Autodesk Inventor part; units mm, degrees
ref_plane "YZ Plane" through (0, 0, 0) normal (1, 0, 0) x (0, 1, 0)
ref_plane "XZ Plane" through (0, 0, 0) normal (0, 1, 0) x (-1, 0, 0)
ref_plane "XY Plane" through (0, 0, 0) normal (0, 0, 1) x (1, 0, 0)
sketch "Boceto1" plane through (0, 0, 0) normal (0, 0, 1) x (1, 0, 0)
  line L0 (0, 50.8) -> (-20.2, 50.8)
  line L1 (-20.2, 50.8) -> (-20.2, 0)
  line L2 (-20.2, 0) -> (0, 0)
  line L3 (0, 0) -> (0, 50.8)
  dimension "d0" = 50.8
  dimension "d1" = 20.2
extrude "Extrusión1" add sketch "Boceto1" against normal blind 3.4
sketch "Boceto3" plane through (0, 0, 0) normal (0, 0, -1) x (-1, 0, 0)
  line L0 (20.2, 50.8) -> (0, 50.8) construction
  line L1 (0, 50.8) -> (0, 0) construction
  circle A0 centre (10.1, 42.1) radius 2
  line L2 (20.2, 0) -> (20.2, 50.8)
  dimension "d20" = 4
  dimension "d21" = 10.1
  dimension "d23" = 8.7
hole "Agujero3" at (-10.1, 42.1, 0) direction (0, 0, -1) diameter 4 end through all countersink diameter 6 countersink angle 90
sketch "Boceto5" plane through (0, 0, 0) normal (0, 0, -1) x (-1, 0, 0)
  line L0 (10.1, 29.1) -> (10.1, 22.1) construction
  line L1 (15.1, 29.1) -> (15.1, 22.1)
  line L2 (5.1, 22.1) -> (5.1, 29.1)
  arc A0 (15.1, 29.1) -> (5.1, 29.1) centre (10.1, 29.1) ccw
  arc A1 (5.1, 22.1) -> (15.1, 22.1) centre (10.1, 22.1) ccw
  circle A2 centre (10.1, 42.1) radius 3
  line L3 (0, 50.8) -> (0, 0)
  point P0 (10.1, 25.6)
  point P1 (10.1, 17.1)
  point P2 (10.1, 34.1)
  dimension "d31" = 10
  dimension "d32" = 17
  dimension "d34" = 5.1
extrude "Extrusión2" cut sketch "Boceto5" along normal through all contours L1 A1 L2 A0
sketch "Boceto6" plane through (0, 0, -3.4) normal (0, 0, -1) x (-1, 0, 0)
  line L0 (0, 0) -> (20.2, 0)
  line L1 (2.9, 0) -> (2.9, 12.8)
  line L2 (2.9, 12.8) -> (17.3, 12.8)
  line L3 (17.3, 12.8) -> (17.3, 0)
  line L4 (16, 0) -> (16, 11.5)
  line L5 (16, 11.5) -> (4.2, 11.5)
  line L6 (4.2, 11.5) -> (4.2, 0)
  line L7 (0, 50.8) -> (0, 0)
  line L8 (20.2, 0) -> (20.2, 50.8)
  point P0 (4.2, 0)
  point P1 (16, 0)
  dimension "d37" = 12.8
  dimension "d40" = 1.3
  dimension "d50" = 14.4
  dimension "d51" = 2.9
  dimension "d52" = 2.9
extrude "Extrusión3" add sketch "Boceto6" along normal blind 12.7 contours L1 L2 L3 L0 L4 L5 L6
sketch "Boceto7" plane through (0, 0, -3.4) normal (0, 0, -1) x (-1, 0, 0)
  line L0 (16, 11.5) -> (16, 0)
  line L1 (4.2, 11.5) -> (16, 11.5)
  line L2 (16, 11.5) -> (16, 0)
  line L3 (16, 0) -> (4.2, 0)
  line L4 (4.2, 0) -> (4.2, 11.5)
  point P0 (0, 0)
  point P1 (16, 11.5)
extrude "Extrusión4" cut sketch "Boceto7" against normal blind 10
properties part number "PLASTICO" material "Plástico ABS"
Input: part model. Units: mm. Frame: model coordinates. A direction names the side the tool comes from. Coordinates: 2 decimals unless noted, no trailing zeros. Order: outer loops, then holes, each group sorted by start corner. A loop starts at its lowest first (then second) coordinate and runs counter-clockwise, first axis right, second up. Notation, with made-up numbers: (44, 24.25) - (96, 24.25) arc R17 cw to (96, 32.25) - close; hole circle Ø2 at (13.5, 36). An arc over 180 degrees is marked (long way). Put each result on its own line as item: value.
1. Cut plane B-B on x = -10.1. Return the cut outline in (y, z).
Report:
outline: (11.5, -16.1) - (12.8, -16.1) - (12.8, -3.4) - (17.1, -3.4) - (17.1, 0) - (11.5, 0) - close; (34.1, -3.4) - (40.1, -3.4) - (40.1, -1) - (39.1, 0) - (34.1, 0) - close; (44.1, -3.4) - (50.8, -3.4) - (50.8, 0) - (45.1, 0) - (44.1, -1) - close
2. Draft query along Y for faces 5 (the face through (-10, 34.1, -1.7)), 6 (the face through (-17, 0, -6)), 7 (the face through (-4.2, 6, -8)), 8 (the face through (-10, 50.8, -2)). Return one class per face: pulls with the +Y half, pulls with the -Y half, needs draft (parallel to the pull), parting line crosses it, or undercut.
Report:
face 5: undercut
face 6: pulls with the -Y half
face 7: needs draft
face 8: pulls with the +Y half
3. Reachability of faces 1 (the face through (-10, 12.8, -10)), 2 (the face through (-16, 6, -8)), 3 (the face through (-2.9, 6, -10)), 4 (the face through (-15.1, 26, -2)) from +Z, -Z, +X, -X, +Y, -Y: full face, straight path, thin tool, end or side. Return the list, or none.
Report:
face 1: -Z, +X, -X, +Y
face 2: +Z, -Z, -Y
face 3: -Z, +X, +Y, -Y
face 4: +Z, -Z
4. Cut plane C-C on z = -13.25. Return the cut outline in (x, y).
Report:
outline: (-17.3, 0) - (-16, 0) - (-16, 11.5) - (-4.2, 11.5) - (-4.2, 0) - (-2.9, 0) - (-2.9, 12.8) - (-17.3, 12.8) - close
5. Contact query for flat-ended pins moving along their axis: pin 1 Ø4 at (y, z) = (4.5, -11) entering from -X; pin 2 Ø4.5 at (x, y) = (-10.1, 42.1) entering from +Z; pin 3 Ø3.5 at (x, z) = (-10.5, -11.5) entering from -Y. Output: stop coordinate, or through.
Report:
pin 1: stops at x = -17.3
pin 2: stops at z = -0.75
pin 3: stops at y = 11.5
6. Cut plane D-D on y = 42.1. Return the cut outline in (x, z).
Report:
outline: (-20.2, -3.4) - (-12.1, -3.4) - (-12.1, -1) - (-13.1, 0) - (-20.2, 0) - close; (-8.1, -3.4) - (0, -3.4) - (0, 0) - (-7.1, 0) - (-8.1, -1) - close
7. Line query: line 1 along Y through (x, z) = (-10.1, -1.8); line 2 along X through (y, z) = (42.1, -2.55); line 3 along X through (y, z) = (8, -2.5). Output: solid intervals per line, ascending.
Report:
line 1: y = 11.5 to 17.1, 34.1 to 40.1, 44.1 to 50.8
line 2: x = -20.2 to -12.1, -8.1 to 0
line 3: x = -20.2 to -16, -4.2 to 0
8. Cut plane A-A on y = 10. Return the cut outline in (x, z), then the cut area to 3 significant figures.
Report:
outline: (-20.2, -3.4) - (-17.3, -3.4) - (-17.3, -16.1) - (-16, -16.1) - (-16, 0) - (-20.2, 0) - close; (-4.2, -16.1) - (-2.9, -16.1) - (-2.9, -3.4) - (0, -3.4) - (0, 0) - (-4.2, 0) - close
area: 61.6 mm2
